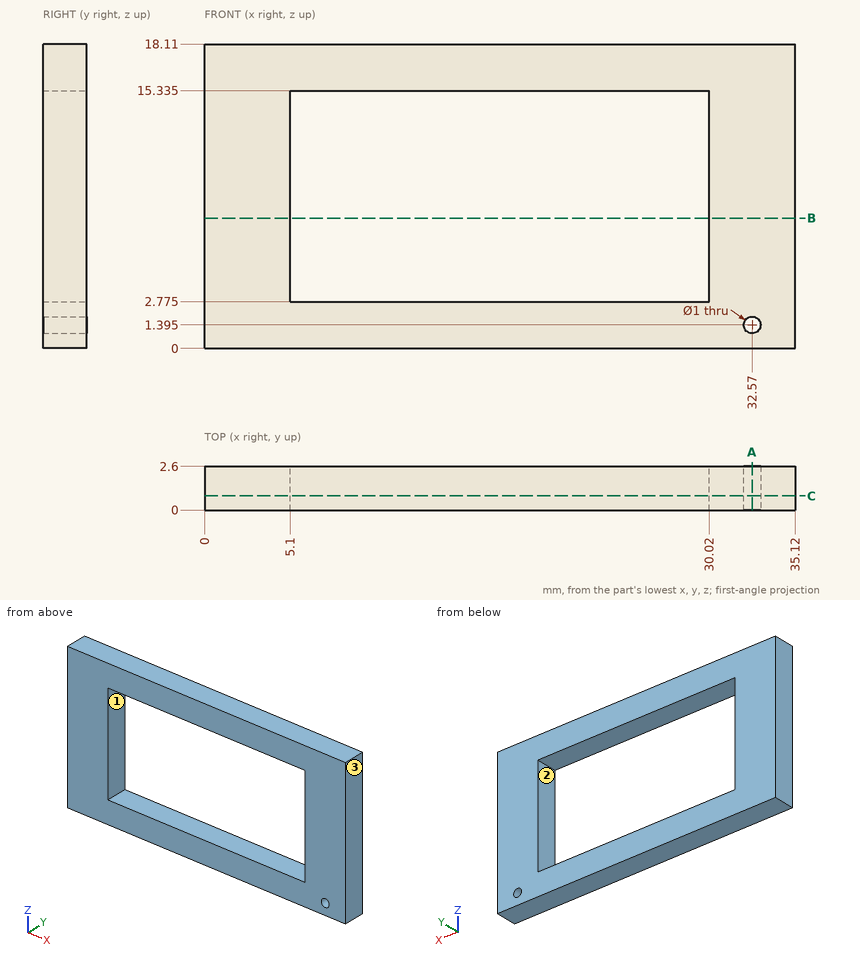
Input: dimensioned drawing with shaded views. Units: mm. Origin: part minimum x, y, z. Give positions to 0.01 mm unless a question says otherwise; leave off trailing zeros. Write each loop counter-clockwise with the first axis right and the second up, starting at its lowest first coordinate (ties: lowest second). Pieces come first, ordered by that corner, then holes.
Q1. Material intervals for probe 1 along X at (y, z) = (1.55, 14.25); probe 2 along Z at (x, y) = (9, 0.25) (3 decimals); probe 3 along Z at (x, y) = (32.57, 1.65) (3 decimals), sorted ascending.
Q2. Section A-A, the plane x = 32.57. Output: boundary loops of the cut face in (y, z) (3 decimals).
Q3. Section C-C, the plane y = 0.85. Output: boundary loops of the cut face in (x, z) (3 decimals), plus the area to 3 significant figures.
Q4. Section B-B, the plane z = 7.75. Output: boundary loops of the cut face in (x, y).
Q5. Pull-direction query (Z, two-part tool) for the marked faces 1, 2 and 3; classes: pulls with the +Z half, pulls with the -Z half, needs draft (parallel to the pull), parting line crosses it, or undercut.
Filled in:
1. probe 1: x = 0 to 5.1, 30.02 to 35.12
1. probe 2: z = 0 to 2.775, 15.335 to 18.11
1. probe 3: z = 0 to 0.895, 1.895 to 18.11
2. outline: (0, 0) - (2.6, 0) - (2.6, 0.895) - (0, 0.895) - close; (0, 1.895) - (2.6, 1.895) - (2.6, 18.11) - (0, 18.11) - close
3. outline: (0, 0) - (35.12, 0) - (35.12, 18.11) - (0, 18.11) - close; hole (5.1, 2.775) - (30.02, 2.775) - (30.02, 15.335) - (5.1, 15.335) - close; hole circle Ø1 at (32.57, 1.395)
3. area: 322 mm2
4. outline: (0, 0) - (5.1, 0) - (5.1, 2.6) - (0, 2.6) - close; (30.02, 0) - (35.12, 0) - (35.12, 2.6) - (30.02, 2.6) - close
5. face 1: undercut
5. face 2: undercut
5. face 3: needs draft
